```python
from build123d import *

# Parameters (mm, degrees)
CROQUIS1_R                 = 16
SALIENTE_EXTRUIR1_DEPTH    = 10
CORTAR_EXTRUIR2_DEPTH      = 10
CORTAR_EXTRUIR4_DEPTH      = 7
CORTAR_EXTRUIR4_DEPTH_BACK = 10
CORTAR_EXTRUIR4_START      = -10
CROQUIS5_R                 = 2
SALIENTE_EXTRUIR2_DEPTH    = 3
CROQUIS6_R                 = 2.8
CROQUIS6_R_2               = 1
SALIENTE_EXTRUIR4_DEPTH    = 2
CORTAR_EXTRUIR5_START      = -12
CROQUIS9_R                 = 1
CORTAR_EXTRUIR5_DEPTH      = 12
CROQUIS10_R                = 6.75
SALIENTE_EXTRUIR5_DEPTH    = 2
CROQUIS11_R                = 6
CORTAR_EXTRUIR6_DEPTH      = 4
CROQUIS12_R                = 0.375
CORTAR_EXTRUIR7_DEPTH      = 7


with BuildPart() as part:
    # Croquis1 → Saliente-Extruir1 (new body)
    with BuildSketch(Plane(origin=(0, 0, 0), x_dir=(1, 0, 0), z_dir=(0, 1, 0))):
        with Locations(Location((0, 0, 0), (0, 0, 270))):
            Circle(CROQUIS1_R)
    extrude(amount=SALIENTE_EXTRUIR1_DEPTH)

    # Croquis2 → Cortar-Extruir2 (cut)
    with BuildSketch(Plane(origin=(0, 0, 0), x_dir=(-1, 0, 0), z_dir=(0, -1, 0))):
        with BuildLine():
            ThreePointArc((-6.5, -14.620191518), (0, -16), (6.5, -14.620191517))
            Line((6.5, -14.620191517), (6.5, -10.035533906))
            Line((6.5, -10.035533906), (4.964466094, -8.5))
            Line((4.964466094, -8.5), (-4.964466094, -8.5))
            Line((-4.964466094, -8.5), (-6.5, -10.035533906))
            Line((-6.5, -10.035533906), (-6.5, -14.620191517))
        make_face()
        with BuildLine():
            Line((-4.964466094, 8.5), (4.964466094, 8.5))
            Line((4.964466094, 8.5), (6.5, 10.035533906))
            Line((6.5, 10.035533906), (6.5, 14.620191517))
            ThreePointArc((6.5, 14.620191518), (0, 16.000000001), (-6.5, 14.620191518))
            Line((-6.5, 14.620191517), (-6.5, 10.035533906))
            Line((-6.5, 10.035533906), (-4.964466094, 8.5))
        make_face()
        with BuildLine():
            Line((10.035533906, -6.5), (14.620191517, -6.5))
            ThreePointArc((14.620191515, -6.499999999), (15.651246979, -3.322418977), (15.999999994, 0))
            ThreePointArc((16, 0), (15.651246984, 3.322418978), (14.620191517, 6.5))
            Line((14.620191517, 6.5), (10.035533906, 6.5))
            Line((10.035533906, 6.5), (8.5, 4.964466094))
            Line((8.5, 4.964466094), (8.5, -4.964466094))
            Line((8.5, -4.964466094), (10.035533906, -6.5))
        make_face()
        with BuildLine():
            ThreePointArc((-14.620191518, 6.5), (-16.000000001, 0), (-14.620191518, -6.5))
            Line((-14.620191517, -6.5), (-10.035533906, -6.5))
            Line((-10.035533906, -6.5), (-8.5, -4.964466094))
            Line((-8.5, -4.964466094), (-8.5, 4.964466094))
            Line((-8.5, 4.964466094), (-10.035533906, 6.5))
            Line((-10.035533906, 6.5), (-14.620191517, 6.5))
        make_face()
    extrude(amount=-CORTAR_EXTRUIR2_DEPTH, mode=Mode.SUBTRACT)

    # Croquis4 → Cortar-Extruir4 (cut, two sides: drawn at the far end of the back side and taken through both)
    with BuildSketch(Plane.XZ.offset(CORTAR_EXTRUIR4_START - CORTAR_EXTRUIR4_DEPTH_BACK)):
        Polygon((-6.5, 16.599431938), (-6.5, 6.5), (-19.32076002, 6.5), (-19.32076002, -6.5), (-6.5, -6.5), (-6.5, -17.296221808), (6.5, -17.296221808), (6.5, -6.5), (20.964302933, -6.5), (20.964302933, 6.5), (6.5, 6.5), (6.5, 16.599431938), align=None)
    extrude(amount=CORTAR_EXTRUIR4_DEPTH + CORTAR_EXTRUIR4_DEPTH_BACK, mode=Mode.SUBTRACT)

    # Croquis5 → Saliente-Extruir2 (add)
    with BuildSketch(Plane(origin=(0, 3, 0), x_dir=(1, 0, 0), z_dir=(0, 1, 0))):
        with Locations(Location((0, 0, 0), (0, 0, 270))):
            Circle(CROQUIS5_R)
    extrude(amount=SALIENTE_EXTRUIR2_DEPTH)

    # Croquis6 → Saliente-Extruir4 (add)
    # profile 1 of 4: a face of its own
    with BuildSketch(Plane(origin=(0, 10, 0), x_dir=(1, 0, 0), z_dir=(0, 1, 0))):
        with Locations(Location((-9.298454173, -9.298454173, 0), (0, 0, 88.096034402))):
            Circle(CROQUIS6_R)
        with Locations(Location((-9.298454173, -9.298454173, 0), (0, 0, 270))):
            Circle(CROQUIS6_R_2, mode=Mode.SUBTRACT)
    # profile 2 of 4: a face of its own
    with BuildSketch(Plane(origin=(0, 10, 0), x_dir=(1, 0, 0), z_dir=(0, 1, 0))):
        with Locations(Location((-9.298454173, 9.298454173, 0), (0, 0, 1.903965598))):
            Circle(CROQUIS6_R)
        with Locations(Location((-9.298454173, 9.298454173, 0), (0, 0, 270))):
            Circle(CROQUIS6_R_2, mode=Mode.SUBTRACT)
    # profile 3 of 4: a face of its own
    with BuildSketch(Plane(origin=(0, 10, 0), x_dir=(1, 0, 0), z_dir=(0, 1, 0))):
        with BuildLine():
            ThreePointArc((9.391482361, 6.5), (11.310974847, 7.351723442), (12.098454173, 9.298454173))
            ThreePointArc((12.098454173, 9.298454173), (9.344974688, 12.098067689), (6.5, 9.391482361))
            Line((6.5, 9.391482361), (6.5, 9.205425984))
            ThreePointArc((6.5, 9.205425984), (7.318555185, 7.318555185), (9.205425984, 6.5))
            Line((9.205425984, 6.5), (9.391482361, 6.5))
        make_face()
        with Locations(Location((9.298454173, 9.298454173, 0), (0, 0, 270))):
            Circle(CROQUIS6_R_2, mode=Mode.SUBTRACT)
    # profile 4 of 4: a face of its own
    with BuildSketch(Plane(origin=(0, 10, 0), x_dir=(1, 0, 0), z_dir=(0, 1, 0))):
        with Locations(Location((9.298454173, -9.298454173, 0), (0, 0, 91.903965598))):
            Circle(CROQUIS6_R)
        with Locations(Location((9.298454173, -9.298454173, 0), (0, 0, 270))):
            Circle(CROQUIS6_R_2, mode=Mode.SUBTRACT)
    extrude(amount=SALIENTE_EXTRUIR4_DEPTH)

    # Croquis9 → Cortar-Extruir5 (cut)
    with BuildSketch(Plane(origin=(0, 10, 0), x_dir=(1, 0, 0), z_dir=(0, 1, 0)).offset(CORTAR_EXTRUIR5_START)):
        with Locations(Location((-9.298454173, 9.298454173, 0), (0, 0, 270))):
            Circle(CROQUIS9_R)
        with Locations(Location((9.298454173, 9.298454173, 0), (0, 0, 270))):
            Circle(CROQUIS9_R)
        with Locations(Location((9.298454173, -9.298454173, 0), (0, 0, 270))):
            Circle(CROQUIS9_R)
        with Locations(Location((-9.298454173, -9.298454173, 0), (0, 0, 270))):
            Circle(CROQUIS9_R)
    extrude(amount=CORTAR_EXTRUIR5_DEPTH, mode=Mode.SUBTRACT)

    # Croquis10 → Saliente-Extruir5 (add)
    with BuildSketch(Plane.XZ):
        with Locations(Location((0, 0, 0), (0, 0, 90))):
            Circle(CROQUIS10_R)
    extrude(amount=SALIENTE_EXTRUIR5_DEPTH)

    # Croquis11 → Cortar-Extruir6 (cut)
    with BuildSketch(Plane.XZ.offset(2)):
        with Locations(Location((0, 0, 0), (0, 0, 270))):
            Circle(CROQUIS11_R)
    extrude(amount=-CORTAR_EXTRUIR6_DEPTH, mode=Mode.SUBTRACT)

    # Croquis12 → Cortar-Extruir7 (cut)
    with BuildSketch(Plane.XZ.offset(2)):
        with Locations(Location((0, 0, 0), (0, 0, 270))):
            Circle(CROQUIS12_R)
    extrude(amount=-CORTAR_EXTRUIR7_DEPTH, mode=Mode.SUBTRACT)


solid = part.part
```
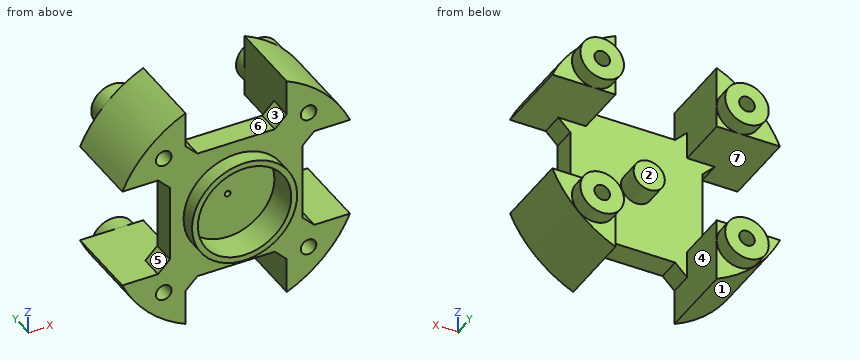
Model file for the job. Use its own axes, mm. Face numbers are marked on the shaded views. A direction names the side the tool comes from. Coordinates: 2 decimals unless noted, no trailing zeros. Loops run counter-clockwise (first coordinate to the right, second up) from the corner with the lowest first, then second, coordinate; pieces in that order, holes last. Notation, with made-up numbers: (77.5, -5.5) - (97.5, -5.5) arc R12 ccw to (97.5, -0.5) - close; hole circle Ø6 at (61, -16). An arc over 180 degrees is marked (long way). Answer as a JSON object with one key per item and string values. Group by question number.
(1) Cut at A-A (y = 9). Give the cut face in (x, z).
(2) Flat gauge pins, fed straight in: pin 1 (1.5 mm diameter, centred on y = 1, z = -1.5, fed in from +X); pin 2 (6 mm diameter, centred on y = 3, z = 10.5, fed in from -X); pin 3 (2 mm diameter, centred on y = 3, z = 5, fed in from -X); pin 4 (1.6 mm diameter, centred on x = -9.3, z = 9.3, fed in from +Y). Where does each tip first touch, or does it go through?
(3) Two-plate mould, pull along X, no slides. Class the marked faces 1, 2 and 3: released by +X, released by -X, zero draft, split by the parting line, or undercut.
(4) Cut at D-D (z = 11). Give the cut face in (x, y), then the cut area to 3 significant figures.
(5) Cut at B-B (x = 0). Give the cut face in (y, z) (3 decimals).
(6) Tool access for the marked faces 4, 5, 6 and 7: list every direction of +Z, -Z, +X, -X, +Y, -Y with a clear straight run to the whole face (end or side of a thin tool).
(7) Cut at C-C (z = 0). Give the cut face in (x, y) (3 decimals), then the cut area to 4 significant figures.
(8) Probe line 1 along X through (y, z) = (9.25, -12.25); line 2 along X through (y, z) = (3.5, -12). List the from-to ranges inside material, lowest first.
Geometry says:
{
 "1": {"outline": "(-14.62, -6.5) arc R16 ccw to (-6.5, -14.62) - (-6.5, -6.5) - close; (-14.62, 6.5) - (-6.5, 6.5) - (-6.5, 14.62) arc R16 ccw to start; (6.5, -14.62) arc R16 ccw to (14.62, -6.5) - (6.5, -6.5) - close; (6.5, 6.5) - (14.62, 6.5) arc R16 ccw to (6.5, 14.62) - close; hole circle Ø2 at (-9.3, -9.3); hole circle Ø2 at (-9.3, 9.3); hole circle Ø2 at (9.3, -9.3); hole circle Ø2 at (9.3, 9.3)"},
 "2": {"pin 1": "stops at x = 8.5", "pin 2": "stops at x = -14.13", "pin 3": "stops at x = -9.54", "pin 4": "passes through"},
 "3": {"face 1": "released by -X", "face 2": "zero draft", "face 3": "undercut"},
 "4": {"outline": "(-11.62, 0) - (-6.5, 0) - (-6.5, 10) - (-7.07, 10) - (-7.07, 12) - (-11.52, 12) - (-11.52, 10) - (-11.62, 10) - close; (6.5, 0) - (11.62, 0) - (11.62, 10) - (11.52, 10) - (11.52, 12) - (7.07, 12) - (7.07, 10) - (6.5, 10) - close", "area": "120 mm^2"},
 "5": {"outline": "(-2, -6.75) - (0, -6.75) - (0, -8.5) - (3, -8.5) - (3, -2) - (6, -2) - (6, 2) - (3, 2) - (3, 8.5) - (0, 8.5) - (0, 6.75) - (-2, 6.75) - (-2, 6) - (2, 6) - (2, 0.375) - (5, 0.375) - (5, -0.375) - (2, -0.375) - (2, -6) - (-2, -6) - close"},
 "6": {"face 4": "-Z, +Y", "face 5": "-X, +Y, -Y", "face 6": "+Z, +Y, -Y", "face 7": "-X, +Y"},
 "7": {"outline": "(-8.5, 0) - (-6.75, 0) - (-6.75, -2) - (-6, -2) - (-6, 2) - (-0.375, 2) - (-0.375, 5) - (0.375, 5) - (0.375, 2) - (6, 2) - (6, -2) - (6.75, -2) - (6.75, 0) - (8.5, 0) - (8.5, 3) - (2, 3) - (2, 6) - (-2, 6) - (-2, 3) - (-8.5, 3) - close", "area": "39.75 mm^2"},
 "8": {"line 1": "x = -10.29 to -6.5, 6.5 to 10.29", "line 2": "x = -10.58 to -6.5, 6.5 to 10.58"}
}
